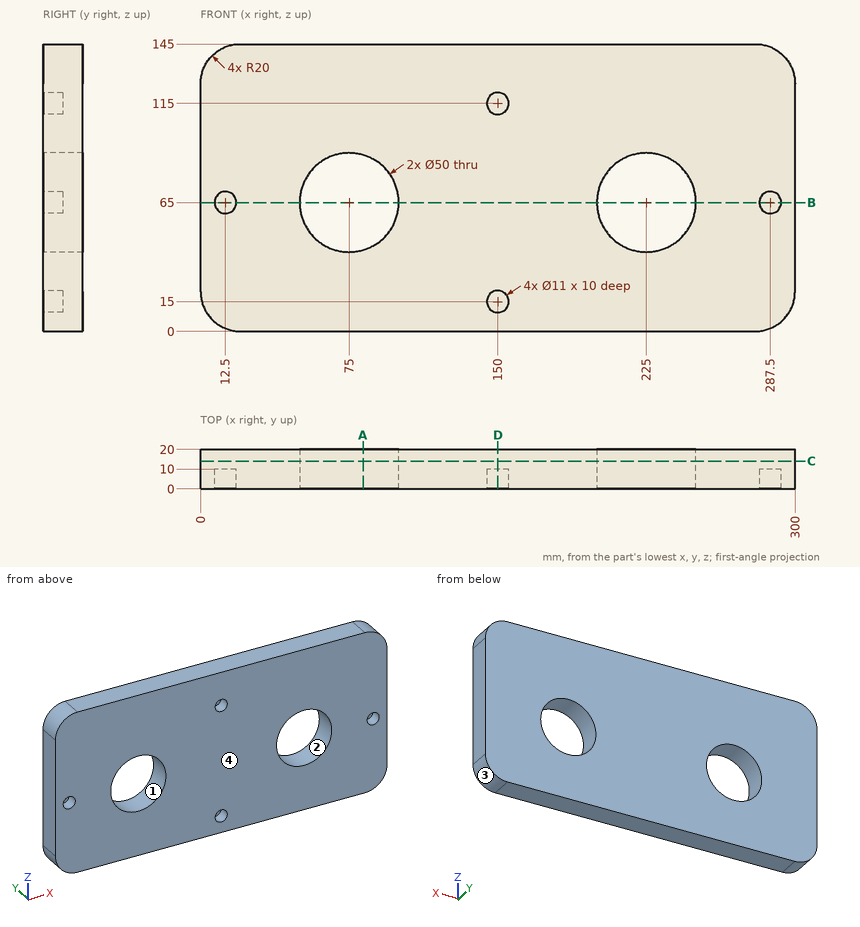
Here's the drawing with two shaded views (mm, measured from the low corner). I have some questions. Give positions to 0.01 mm unless a question says otherwise; leave off trailing zeros. Write each loop counter-clockwise with the first axis right and the second up, starting at its lowest first coordinate (ties: lowest second). Pieces come first, ordered by that corner, then holes. Notation, with made-up numbers: (62, 4.25) - (111, 4.25) arc R22 ccw to (111, 29.25) - close; hole circle Ø9 at (-15.75, -1.5). An arc over 180 degrees is marked (long way). Write item = value, one per line. Start each with the question number.
1. Imagine slicing it at D-D (x = 150). Please give me the cut outline in (y, z).
2. Imagine slicing it at C-C (y = 14). Please give me the cut outline in (x, z), and give its area (3 significant figures).
3. Thinking about a two-plate mould opening in X: for the marked faces 1, 2, 3 and 4, which applies, released by +X, released by -X, zero draft, split by the parting line, or undercut?
4. Imagine slicing it at B-B (z = 65). Please give me the cut outline in (x, y), and give its area (3 significant figures).
5. Imagine slicing it at A-A (x = 82). Please give me the cut outline in (y, z), and give its area (3 significant figures).
6. Please list where these lines run through material, in increasing order: line 1 (X direction, y = 7.75, z = 53.5); line 2 (Z direction, x = 75, y = 13.75); line 3 (X direction, y = 11, z = 80).
7. For pin 1 (3.5 mm diameter, centred on x = 148.5, z = 115, fed in from -Y); pin 2 (1 mm diameter, centred on y = 9.5, z = 18.5, fed in from -X) (3 decimals), each with a flat end and sliding along its axis, tell me the tip position at first contact or that it passes through.
Worked answers:
q1.outline = (0, 0) - (20, 0) - (20, 145) - (0, 145) - (0, 120.5) - (10, 120.5) - (10, 109.5) - (0, 109.5) - (0, 20.5) - (10, 20.5) - (10, 9.5) - (0, 9.5) - close
q2.outline = (0, 20) arc R20 ccw to (20, 0) - (280, 0) arc R20 ccw to (300, 20) - (300, 125) arc R20 ccw to (280, 145) - (20, 145) arc R20 ccw to (0, 125) - close; hole circle Ø50 at (75, 65); hole circle Ø50 at (225, 65)
q2.area = 39,200 mm2
q3.face_1 = undercut
q3.face_2 = undercut
q3.face_3 = released by +X
q3.face_4 = zero draft
q4.outline = (0, 0) - (7, 0) - (7, 10) - (18, 10) - (18, 0) - (50, 0) - (50, 20) - (0, 20) - close; (100, 0) - (200, 0) - (200, 20) - (100, 20) - close; (250, 0) - (282, 0) - (282, 10) - (293, 10) - (293, 0) - (300, 0) - (300, 20) - (250, 20) - close
q4.area = 3,780 mm2
q5.outline = (0, 0) - (20, 0) - (20, 41) - (0, 41) - close; (0, 89) - (20, 89) - (20, 145) - (0, 145) - close
q5.area = 1,940 mm2
q6.line_1 = 0 to 52.8, 97.2 to 202.8, 247.2 to 300
q6.line_2 = 0 to 40, 90 to 145
q6.line_3 = 0 to 55, 95 to 205, 245 to 300
q7.pin_1 = 10
q7.pin_2 = 0.025
